```python
from build123d import *

# Parameters (mm, degrees)
F1_R          = 21
F3_DEPTH      = 21.0010001
F3_DEPTH_BACK = 21.0010001


with BuildPart() as f2:
    # F2: sweep along a path in F0
    with BuildLine(Plane.XZ) as f2_path:
        Line((0, 0), (0, -199.5701125716))
        ThreePointArc((0, -199.5701125716), (-12.7613665352, -241.419276296), (-46.7027334515, -269.0270395543))
        Line((-46.7027334515, -269.0270395543), (-216, -338))
    # F1 (on Top) → F2 (sweep)
    with BuildSketch(Plane.XY):
        Circle(F1_R)
    sweep(path=f2_path.line)

    # F0 (on Front) → F3 (cut, two sides)
    with BuildSketch(Plane.XZ) as f3_sk:
        with BuildLine():
            ThreePointArc((0, -30.15), (21.3192694528, -21.3192694528), (30.15, 0))
            ThreePointArc((30.15, 0), (-21.3192694528, 21.3192694528), (0, -30.15))
        make_face()
        with BuildLine():
            ThreePointArc((-191.87, -338), (-192.3200446948, -333.3613992688), (-193.6533913588, -328.8958261091))
            ThreePointArc((-193.6533913588, -328.8958261091), (-239.6799553052, -342.6386007312), (-191.87, -338))
        make_face()
    extrude(amount=-F3_DEPTH, mode=Mode.SUBTRACT)
    extrude(f3_sk.sketch, amount=F3_DEPTH_BACK, mode=Mode.SUBTRACT)


solid = f2.part
```
Here's how the part is built. I have some questions about the finished solid (model axes, mm). A direction names the side the tool comes from. Give positions to 0.01 mm unless a question says otherwise; leave off trailing zeros. Loops run counter-clockwise (first coordinate to the right, second up) from the corner with the lowest first, then second, coordinate; pieces in that order, holes last. Notation, with made-up numbers: (33.25, 31) -> (64.25, 31) arc R15 cw to (64.25, 47) -> close; hole circle Ø8 at (68, 11.25). An arc over 180 degrees is marked (long way). Use one line per item in the form item = value. Start each with the question number.
1) Imagine slicing it at B-B (z = -45). Please give me the cut outline in (x, y), then the cut area to 3 significant figures.
2) Imagine slicing it at C-C (y = -11). Please give me the cut outline in (x, z), then the cut area to 3 significant figures.
3) Which directions (+Z, -Z, +X, -X, +Y, -Y) give clear straight access to the entire face, cutting with the end or side of a thin tool? Please do faces 1 (the face through (20.03, -6.31, -111.85)), 2 (the face through (-134.872, -0.923, -282.294)).
4) Please list where these lines run through material, in increasing order: line 1 along Y through (x, z) = (-31.5, -244); line 2 along X through (y, z) = (-6, -292.5); line 3 along Z through (x, y) = (-149.5, 0).
5) For P1, Ø5, axis at x = -137.5, y = -9, coming from the +Z side; P2, Ø1, axis at y = -10, z = -193.5, coming from the +X side; P3, Ø8, axis at y = -8.5, z = -219, coming from the -X side, each with a flat end and sliding along its axis, tell me the tip position at first contact or that it passes through.
6) Imagine slicing it at A-A (y = 5). Please give me the cut outline in (x, z).
Check values:
q1.outline = circle Ø42 at (0, 0)
q1.area = 1,390 mm^2
q2.outline = (-207.75, -315.32) arc R24.13 cw to (-194.25, -348.46) -> (-39.95, -285.59) arc R92.89 ccw to (17.89, -199.57) -> (17.89, -24.27) arc R30.15 cw to (-17.89, -24.27) -> (-17.89, -199.57) arc R57.11 cw to (-53.45, -252.46) -> close
q2.area = 15,100 mm^2
q3.face_1 = +Z
q3.face_2 = none
q4.line_1 = -16.63 to 16.63
q4.line_2 = -157.66 to -50.98
q4.line_3 = -333.58 to -288.23
q5.P1 = -284.01
q5.P2 = 18.73
q5.P3 = -24.98
q6.outline = (-211.75, -314.25) arc R24.13 cw to (-196.36, -352.02) -> (-39.01, -287.92) arc R95.4 ccw to (20.4, -199.57) -> (20.4, -22.2) arc R30.15 cw to (-20.4, -22.2) -> (-20.4, -199.57) arc R54.6 cw to (-54.4, -250.14) -> close
